Design review of the part built by this model. Coordinates are the model's own, in mm. A direction names the side the tool comes from. Give positions to 0.01 mm unless a question says otherwise; leave off trailing zeros. Write each loop counter-clockwise with the first axis right and the second up, starting at its lowest first coordinate (ties: lowest second). Pieces come first, ordered by that corner, then holes. Notation, with made-up numbers: M 10.25,87.5 L 18.25,87.5 A3 cw 18.25,92.5 Z; hole C 25,-25 d8. An arc over 180 degrees is marked long. Answer in a Markdown table with one row per item.
```python
from build123d import *

# Parameters (mm, degrees)
F0_W     = 1.9742772416
F0_H     = 18.7233856638
F0_W_2   = 88.3857645094
F0_W_3   = 1.7149582489
F1_DEPTH = 25.4
F3_D     = 3
F0_H_2   = 510.4961821119
F0_H_3   = 496.8783685247
F4_DEPTH = 25.4


with BuildPart() as f1:
    # F0 (on Top) → F1 (new body)
    with BuildSketch(Plane.XY):
        with Locations((-46.5922877409, 9.3616928319)):
            Rectangle(F0_W, F0_H)
        with Locations((-1.4122668654, 9.3616928319)):
            Rectangle(F0_W_2, F0_H)
        with Locations((43.6380945138, 9.3616928319)):
            Rectangle(F0_W_3, F0_H)
    extrude(amount=-F1_DEPTH)

    # F3 (through all)
    with Locations(Plane.XY):
        with Locations((3.7512294251, 10.0710503428), (-3.3089503626, 10.1887194856), (-12.4521386383, 10.1791908965)):
            Hole(F3_D / 2)

    # F0 (on Top) → F4 (join)
    with BuildSketch(Plane.XY):
        with Locations((-46.5922877409, 273.9714767198)):
            Rectangle(F0_W, F0_H_2)
        with Locations((-46.5922877409, 9.3616928319)):
            Rectangle(F0_W, F0_H)
        with Locations((-1.4122668654, 9.3616928319)):
            Rectangle(F0_W_2, F0_H)
        with Locations((43.6380945138, 267.1625699262)):
            Rectangle(F0_W_3, F0_H_3)
        with Locations((43.6380945138, 9.3616928319)):
            Rectangle(F0_W_3, F0_H)
    extrude(amount=F4_DEPTH)


solid = f1.part
```
1) The part is to be moulded in two halves that separate along X. For faces 3 (the face through (-47.579, 268, 17)), 4 (the face through (42.781, 264, 13)), 5 (the face through (-46, 148, 25.4)), say which applies: released by +X, released by -X, zero draft, split by the parting line, or undercut.
Geometry says:
| item | result |
|---|---|
| face 3 | released by -X |
| face 4 | undercut |
| face 5 | zero draft |
2) Add section B-B (z = -7). Write out the cut boundary in (x, y), and give its area (3 significant figures).
Geometry says:
| item | result |
|---|---|
| outline | M -47.58,0 L 44.5,0 L 44.5,18.72 L -47.58,18.72 Z; hole C -12.45,10.18 d3; hole C -3.31,10.19 d3; hole C 3.75,10.07 d3 |
| area | 1,700 mm^2 |
3) Add section C-C (z = 19.5). Write out the cut boundary in (x, y), and give its area (3 significant figures).
Geometry says:
| item | result |
|---|---|
| outline | M -47.58,0 L 44.5,0 L 44.5,515.6 L 42.78,515.6 L 42.78,18.72 L -45.61,18.72 L -45.61,529.22 L -47.58,529.22 Z |
| area | 3,580 mm^2 |
4) To check wall thickness, follow probe 1 along X at (y, z) = (356, 20.5); probe 2 along Y at (x, z) = (12, -6). State the ranges of each line that lie inside material, in increasing order. Write a range as [from, to].
Geometry says:
| item | result |
|---|---|
| probe 1 | [-47.58, -45.61], [42.78, 44.5] |
| probe 2 | [0, 18.72] |
5) Insertion check: P1, Ø0.9, axis at x = 43.5, y = 156, coming from the -Z side; P2, Ø0.9, axis at x = 43.5, z = 7.5, coming from the +Y side; P3, Ø8, axis at x = -12.5, z = 7, coming from the +Y side. Each pin has a flat end and moves straight along its axis. Give the tip position at first contact, or say it passes through.
Geometry says:
| item | result |
|---|---|
| P1 | z = 0 |
| P2 | y = 515.6 |
| P3 | y = 18.72 |
6) For faces 1 (the face through (-2, 0, 0)), 2 (the face through (-45.605, 270, 13)), list the 3-axis set-ups (+Z, -Z, +X, -X, +Y, -Y) from which the entire face can be reached by the end or side of a thin tool; tool diameter is ignored.
Geometry says:
| item | result |
|---|---|
| face 1 | +Z, -Z, +X, -X, -Y |
| face 2 | +Z, -Z, +Y |
7) Add section A-A (y = 384.5). Write out the cut boundary in (x, z).
Geometry says:
| item | result |
|---|---|
| outline | M -47.58,0 L -45.61,0 L -45.61,25.4 L -47.58,25.4 Z; M 42.78,0 L 44.5,0 L 44.5,25.4 L 42.78,25.4 Z |
8) Add section D-D (x = -35). Write out the cut boundary in (y, z), and give its area (3 significant figures).
Geometry says:
| item | result |
|---|---|
| outline | M 0,-25.4 L 18.72,-25.4 L 18.72,25.4 L 0,25.4 Z |
| area | 951 mm^2 |
